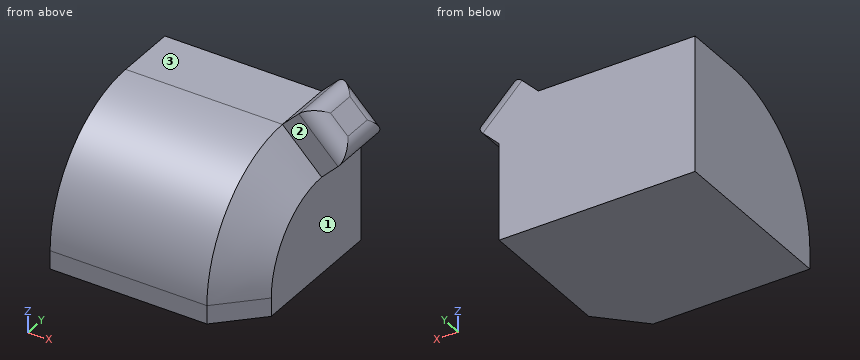
```python
from build123d import *

# Parameters (mm, degrees)
F0_W     = 127
F0_H     = 115.7713381711
F1_DEPTH = 88.138
F2_R     = 76.2
F3_SIZE  = 25.4
F4_DEPTH = 25
F5_R     = 10


# Not quite as in the source:
# - a feature of the source that left no trace in its solid (it failed there, or was rolled back) is left out


with BuildPart() as f1:
    # F0 (on Top) → F1 (new body)
    with BuildSketch(Plane.XY):
        with Locations((0.6131026894, 1.0218378156)):
            Rectangle(F0_W, F0_H)
    extrude(amount=F1_DEPTH)

    # F2
    f2_edges = [f1.edges().sort_by_distance(p)[0] for p in [
        (0.613103, -56.863831, 88.138),
    ]]
    fillet(f2_edges, radius=F2_R)

    # F3
    f3_edges = [f1.edges().sort_by_distance(p)[0] for p in [
        (64.113103, 39.121838, 88.138),
        (64.113103, -56.863831, 5.969),
        (64.113103, -34.545368, 65.819537),
    ]]
    chamfer(f3_edges, length=F3_SIZE)

    # F4 (add): a face of the model
    f4_faces = [f1.faces().sort_by_distance(p)[0] for p in [
        (51.4131026894, 39.1218378156, 75.438),
    ]]
    extrude(f4_faces, amount=F4_DEPTH)

    # F5
    f5_edges = [f1.edges().sort_by_distance(p)[0] for p in [
        (69.090772, 58.907507, 93.11567),
        (69.090772, 19.336169, 93.11567),
        (56.390772, 39.121838, 105.81567),
        (81.790772, 39.121838, 80.41567),
    ]]
    fillet(f5_edges, radius=F5_R)


solid = f1.part
```
Can you work these out from the model? Positions are in its coordinate system, mm. Face numbers are marked on the shaded views. A direction names the side the tool comes from. Give positions to 0.01 mm unless a question says otherwise; leave off trailing zeros. Loops run counter-clockwise (first coordinate to the right, second up) from the corner with the lowest first, then second, coordinate; pieces in that order, holes last. Notation, with made-up numbers: M -22.75,-18 L 23.25,-18 A19 cw 23.25,9 Z; hole C 50.5,24 d2. An arc over 180 degrees is marked long. Use CSV: the item, a comma, the result in double quotes. Start each with the question number.
1. If I drill on L1, parallel to X at y = 37.5, z = 40; L2, parallel to Z at x = -36, y = 37; L3, parallel to Y at x = -10.5, z = 14, over which ranges is the centre line in solid material (lowest first)?
2. On a 3-axis mill with a long thin cutter (end or side, diameter ignored), from which of +Z, -Z, +X, -X, +Y, -Y can I reach the whole of each face in a straight line? I mean the marked faces 1, 2 and 3. Say none if no direction works.
3. Imagine slicing it at C-C, the plane x = 41. Write out the boundary of the cut face in (y, z).
4. Imagine slicing it at B-B, the plane x = 16. Write out the boundary of the cut face in (y, z), plus the area to 3 significant figures.
5. Imagine slicing it at A-A, the plane y = 33.5. Write out the boundary of the cut face in (x, z).
6. For P1, Ø3, axis at x = 61.5, z = 89, coming from the +Y side; P2, Ø6, axis at x = -30.5, y = 24, coming from the +Z side; P3, Ø10, axis at x = -17.5, y = -41.5, coming from the -Z side; P4, Ø12, axis at x = -40.5, y = -9.5, coming from the +Z side, each with a flat end and sliding along its axis, tell me the tip position at first contact or that it passes through.
Response values:
1,L1,"-62.89 to 64.11"
1,L2,"0 to 88.14"
1,L3,"-56.84 to 58.91"
2,face 1,"-Z, +X, +Y, -Y"
2,face 2,"+Z, +X, -Y"
2,face 3,"+Z, -X, +Y, -Y"
3,outline,"M -54.58,0 L 58.91,0 L 58.91,90.42 L 19.34,90.42 L 19.34,85.85 A73.91 ccw -54.58,11.94 Z"
4,outline,"M -56.86,0 L 58.91,0 L 58.91,88.14 L 19.34,88.14 A76.2 ccw -56.86,11.94 Z"
4,area,"8,960 mm^2"
5,outline,"M -62.89,0 L 64.11,0 L 64.11,62.74 L 74.72,73.34 A10 ccw 74.72,87.49 L 63.46,98.74 A10 ccw 49.32,98.74 L 38.71,88.14 L -62.89,88.14 Z"
6,P1,"y = 58.91"
6,P2,"z = 88.14"
6,P3,"z = 0"
6,P4,"z = 84.64"
